Read the model definition and answer for the solid it produces. Units are mm, in the model's axes. A direction names the side the tool comes from. Give positions to 0.01 mm unless a question says otherwise; leave off trailing zeros. Loops run counter-clockwise (first coordinate to the right, second up) from the corner with the lowest first, then second, coordinate; pieces in that order, holes last. Notation, with made-up numbers: (-21, 46) - (10, 46) arc R19 ccw to (10, 82) - close; hole circle Ø11 at (28.25, 35). An arc over 180 degrees is marked (long way). Use a Markdown table: item, result. Add a question column.
Item 1: For a pull along Z with two mould halves and no side action, classify faces 1 (the face through (-1, 26, -50.8)), 2 (the face through (14.3, 9.9, 11.2)), 3 (the face through (-12.7, 11, -1)), 4 (the face through (-14.27, 12.84, 41.27)) as +Z half, -Z half, draft (parallel to the pull), parting line (faces both ways), or undercut.
Item 2: A cutting plane is placed at C-C (z = 20.5). Determine the outline of the cut face in (x, y) (3 decimals).
Item 3: Which of the six approach directions +Z, -Z, +X, -X, +Y, -Y give full straight-line access (tool end or side, diameter ignored) to faces 5 (the face through (0, 28.702, -1)), 6 (the face through (12.7, 11, -1))?
Item 4: A cutting plane is placed at D-D (y = 12.7). Give the number of separate pieces and of enclosed holes in the cut face, plus the area to 3 significant figures.
Item 5: A cutting plane is placed at A-A (z = -12.7). Determine the outline of the cut face in (x, y) (3 decimals), plus the area to 3 significant figures.
Item 6: A cutting plane is placed at B-B (y = 7). Determine the outline of the cut face in (x, z) (3 decimals).
Item 7: Consider probe 1 along X at (y, z) = (8.75, -16) (3 decimals); probe 2 along Y at (x, z) = (5, -1); probe 3 along X at (y, z) = (24.75, -38.5) (3 decimals). Determine where each line is inside the solid, lowest interval first. Write a range as [from, to].
Item 8: Each of these flat-tipped pins is pushed along its axis until it touches: P1, Ø5, axis at x = 6, z = 25.5, coming from the -Y side; P2, Ø5, axis at y = 12.7, z = -38.1, coming from the +X side; P3, Ø15, axis at x = -4, z = -23.5, coming from the -Y side. Where does it stop, or does it pass through?
Autodesk Inventor part; units mm, degrees
ref_plane "YZ Plane" through (0, 0, 0) normal (1, 0, 0) x (0, 1, 0)
ref_plane "XZ Plane" through (0, 0, 0) normal (0, 1, 0) x (-1, 0, 0)
ref_plane "XY Plane" through (0, 0, 0) normal (0, 0, 1) x (1, 0, 0)
sketch "Sketch1" plane through (0, 0, 0) normal (0, 0, 1) x (1, 0, 0)
  line L0 (-15.875, 0) -> (-12.7, 0)
  line L1 (-12.7, 0) -> (-12.7, 22.352)
  line L2 (-9.525, 25.527) -> (9.525, 25.527)
  line L3 (12.7, 22.352) -> (12.7, 0)
  line L4 (12.7, 0) -> (15.875, 0)
  line L5 (15.875, 0) -> (15.875, 25.527)
  line L6 (12.7, 28.702) -> (-12.7, 28.702)
  line L7 (-15.875, 25.527) -> (-15.875, 0)
  arc A0 (-9.525, 25.527) -> (-12.7, 22.352) centre (-9.525, 22.352) ccw
  arc A1 (12.7, 22.352) -> (9.525, 25.527) centre (9.525, 22.352) ccw
  arc A2 (-12.7, 28.702) -> (-15.875, 25.527) centre (-12.7, 25.527) ccw
  arc A3 (15.875, 25.527) -> (12.7, 28.702) centre (12.7, 25.527) ccw
  line L8 (0, 35.2315) -> (0, -5.8719)
  point P0 (0, 0)
  dimension "d0" = 28.702
  dimension "d1" = 31.75
  dimension "d2" = 3.175
  dimension "d3" = 3.175
  dimension "d4" = 3.175
extrude "Extrusion1" add sketch "Sketch1" along normal mid plane 101.6
sketch "Sketch4" plane through (15.875, 0, 50.8) normal (1, 0, 0) x (0, 0, -1)
  line L0 (50.8, -5.7404) -> (50.8, 34.4424) construction
  line L1 (-33.655, 0) -> (201.93, 0) construction
  circle A0 centre (63.5, 12.7) radius 3.175
  point P0 (50.8, 0)
  dimension "d34" = 12.7
  dimension "d35" = 12.7
  dimension "d36" = 6.35
extrude "Extrusion4" cut sketch "Sketch4" against normal up to surface (31.75 mm away)
pattern_linear "Rectangular Pattern3" count 30 spacing 25.4 along (0, 0, 1) count 30 spacing 25.4 along (0, 0, -1) of "Extrusion4"
equation "\"d5\" = ExtensionLen"
equation "\"ExtensionLen\" = 101.6"
properties part number "NTowerChannelMotor" material "Aluminum 6061"
Geometry says:
| question | item | result |
|---|---|---|
| 1 | face 1 | -Z half |
| 1 | face 2 | undercut |
| 1 | face 3 | draft |
| 1 | face 4 | undercut |
| 2 | outline | (-15.875, 0) - (-12.7, 0) - (-12.7, 22.352) arc R3.175 cw to (-9.525, 25.527) - (9.525, 25.527) arc R3.175 cw to (12.7, 22.352) - (12.7, 0) - (15.875, 0) - (15.875, 25.527) arc R3.175 ccw to (12.7, 28.702) - (-12.7, 28.702) arc R3.175 ccw to (-15.875, 25.527) - close |
| 3 | face 5 | +Z, -Z, +X, -X, +Y |
| 3 | face 6 | +Z, -Z, -Y |
| 4 | separate pieces | 10 |
| 4 | enclosed holes | 0 |
| 4 | area | 484 mm² |
| 5 | outline | (-15.875, 0) - (-12.7, 0) - (-12.7, 9.525) - (-15.875, 9.525) - close; (-15.875, 15.875) - (-12.7, 15.875) - (-12.7, 22.352) arc R3.175 cw to (-9.525, 25.527) - (9.525, 25.527) arc R3.175 cw to (12.7, 22.352) - (12.7, 15.875) - (15.875, 15.875) - (15.875, 25.527) arc R3.175 ccw to (12.7, 28.702) - (-12.7, 28.702) arc R3.175 ccw to (-15.875, 25.527) - close; (12.7, 0) - (15.875, 0) - (15.875, 9.525) - (12.7, 9.525) - close |
| 5 | area | 223 mm² |
| 6 | outline | (-15.875, -50.8) - (-12.7, -50.8) - (-12.7, 50.8) - (-15.875, 50.8) - close; (12.7, -50.8) - (15.875, -50.8) - (15.875, 50.8) - (12.7, 50.8) - close |
| 7 | probe 1 | [-15.875, -12.7], [12.7, 15.875] |
| 7 | probe 2 | [25.53, 28.7] |
| 7 | probe 3 | [-15.875, -11.606], [11.606, 15.875] |
| 8 | P1 | y = 25.53 |
| 8 | P2 | through |
| 8 | P3 | y = 24.84 |
